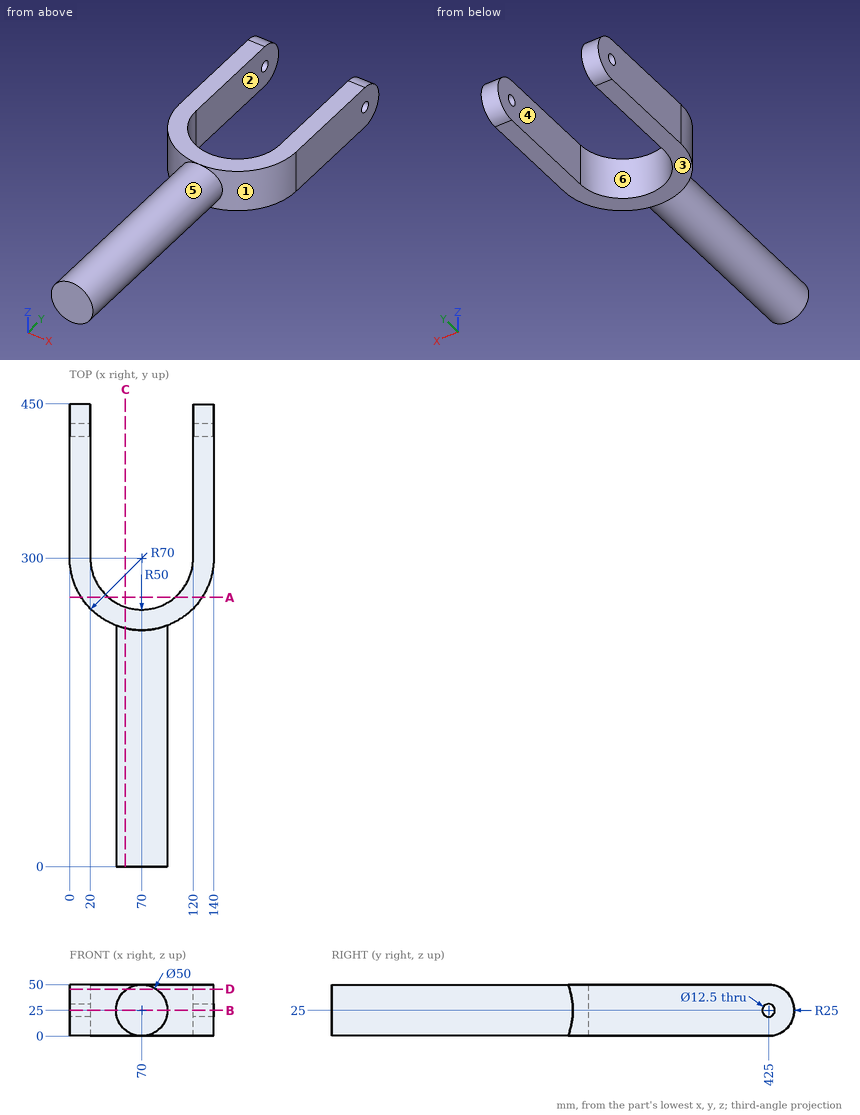
Drawing for the job (mm, zero at the part's lowest x, y, z). A direction names the side the tool comes from. Give positions to 0.01 mm unless a question says otherwise; leave off trailing zeros. Loops run counter-clockwise (first coordinate to the right, second up) from the corner with the lowest first, then second, coordinate; pieces in that order, holes last.
1) 3-axis set-ups, long thin cutter, end or side, ignore diameter. For the marked faces 5 and 6: which of +Z, -Z, +X, -X, +Y, -Y reach the whole face in a straight line?
Values follow:
face 5: -Y
face 6: +Z, -Z, +Y
2) Two-plate mould, pull along X, no slides. Class the marked faces 1, 2, 3 and 4: released by +X, released by -X, zero draft, split by the parting line, or undercut.
Values follow:
face 1: released by +X
face 2: undercut
face 3: zero draft
face 4: undercut
3) Band-saw the part on D-D on z = 45.5. List the corners of the cut face in (x, y), then the cut area to 3 significant figures.
Values follow:
outline: (0, 300) arc R70 ccw to (55.69, 231.48) - (55.69, 0) - (84.31, 0) - (84.31, 231.48) arc R70 ccw to (140, 300) - (140, 439.31) - (120, 439.31) - (120, 300) arc R50 cw to (20, 300) - (20, 439.31) - (0, 439.31) - close
area: 15,900 mm2
4) Probe line 1 along X through (y, z) = (425, 11.5); line 2 along X through (y, z) = (270, 30); line 3 along X through (y, z) = (91.5, 23.5). List the from-to ranges inside material, lowest first.
Values follow:
line 1: x = 0 to 20, 120 to 140
line 2: x = 6.75 to 30, 110 to 133.25
line 3: x = 45.05 to 94.95
5) Band-saw the part on C-C on x = 54. List the corners of the cut face in (y, z), then the cut area to 3 significant figures.
Values follow:
outline: (0, 5.79) - (231.85, 5.79) - (231.85, 0) - (252.63, 0) - (252.63, 50) - (231.85, 50) - (231.85, 44.21) - (0, 44.21) - close
area: 9,950 mm2
6) Band-saw the part on B-B on z = 25. List the corners of the cut face in (x, y), then the cut area to 3 significant figures.
Values follow:
outline: (0, 300) arc R70 ccw to (45, 234.62) - (45, 0) - (95, 0) - (95, 234.62) arc R70 ccw to (140, 300) - (140, 418.75) - (120, 418.75) - (120, 300) arc R50 cw to (20, 300) - (20, 418.75) - (0, 418.75) - close; (0, 431.25) - (20, 431.25) - (20, 450) - (0, 450) - close; (120, 431.25) - (140, 431.25) - (140, 450) - (120, 450) - close
area: 20,800 mm2
7) Drop flat-ended pins along their axis: P1, Ø4, axis at x = 75.5, y = 150.5, coming from the +Z side; P2, Ø4, axis at x = 49.5, y = 182.5, coming from the +Z side; P3, Ø11, axis at y = 425, z = 25, coming from the +X side; P4, Ø8, axis at x = 61, y = 56.5, coming from the +Z side. Give the stop position or say it passes through.
Values follow:
P1: stops at z = 49.75
P2: stops at z = 41.82
P3: passes through
P4: stops at z = 49.49
8) Band-saw the part on A-A on y = 262. List the corners of the cut face in (x, z), then the cut area to 3 significant figures.
Values follow:
outline: (11.21, 0) - (37.5, 0) - (37.5, 50) - (11.21, 50) - close; (102.5, 0) - (128.79, 0) - (128.79, 50) - (102.5, 50) - close
area: 2,630 mm2
